Verification items for this drawing (mm, ordinates from the low corner). Round coordinates to 2 decimals unless told otherwise and drop trailing zeros. Order: outer loops, then holes, each group sorted by start corner. A loop starts at its lowest first (then second) coordinate and runs counter-clockwise, first axis right, second up. Notation, with made-up numbers: M 37.25,40.5 L 96.25,40.5 A26 cw 96.25,61.5 Z; hole C 14.25,48 d4. An arc over 180 degrees is marked long. Return JSON: item names as keys, results as strings. Group by question number.
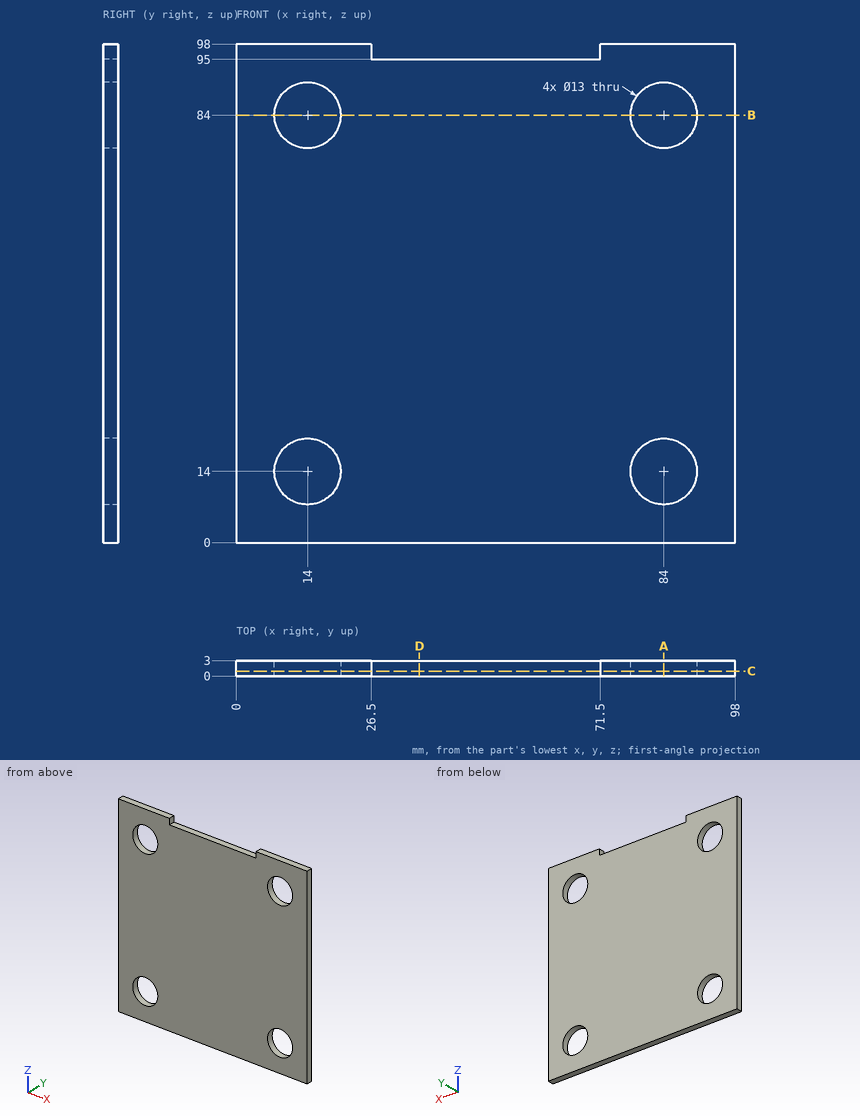
1. Thickness scan on line 1 along Z through (x, y) = (14, 2.4); line 2 along X through (y, z) = (0.4, 78.5); line 3 along X through (y, z) = (1.8, 11.5). Record the ranges inside material, lowest first. Write a range as from..to.
2. Cross-section at B-B (z = 84). Enter the section's corners in (x, y).
3. Cross-section at A-A (x = 84). Enter the section's corners in (y, z).
4. Cross-section at C-C (y = 0.95). Enter the section's corners in (x, z), plus the area to 3 significant figures.
5. Cross-section at D-D (x = 36). Enter the section's corners in (y, z).
6. Go/stop test with flat-tipped pins: pin 1 (10.5 mm diameter, centred on x = 14, z = 14, fed in from +Y); pin 2 (0.9 mm diameter, centred on x = 41.5, y = 2, fed in from +Z). Record where each tip stops, or that it passes through.
Computed:
{
 "1": {"line 1": "z = 0..7.5, 20.5..77.5, 90.5..98", "line 2": "x = 0..10.54, 17.46..80.54, 87.46..98", "line 3": "x = 0..8, 20..78, 90..98"},
 "2": {"outline": "M 0,0 L 7.5,0 L 7.5,3 L 0,3 Z; M 20.5,0 L 77.5,0 L 77.5,3 L 20.5,3 Z; M 90.5,0 L 98,0 L 98,3 L 90.5,3 Z"},
 "3": {"outline": "M 0,0 L 3,0 L 3,7.5 L 0,7.5 Z; M 0,20.5 L 3,20.5 L 3,77.5 L 0,77.5 Z; M 0,90.5 L 3,90.5 L 3,98 L 0,98 Z"},
 "4": {"outline": "M 0,0 L 98,0 L 98,98 L 71.5,98 L 71.5,95 L 26.5,95 L 26.5,98 L 0,98 Z; hole C 14,14 d13; hole C 14,84 d13; hole C 84,14 d13; hole C 84,84 d13", "area": "8,940 mm²"},
 "5": {"outline": "M 0,0 L 3,0 L 3,95 L 0,95 Z"},
 "6": {"pin 1": "passes through", "pin 2": "stops at z = 95"}
}
